Here's the drawing with two shaded views (mm, measured from the low corner). I have some questions. A direction names the side the tool comes from. Round coordinates to 2 decimals unless told otherwise and drop trailing zeros. Loops run counter-clockwise (first coordinate to the right, second up) from the corner with the lowest first, then second, coordinate; pieces in that order, holes last. Notation, with made-up numbers: (57.25, -10) -> (110.25, -10) arc R23 cw to (110.25, 9) -> close; hole circle Ø11 at (48, 64.5). An arc over 180 degrees is marked (long way). Use a Markdown table: item, result.
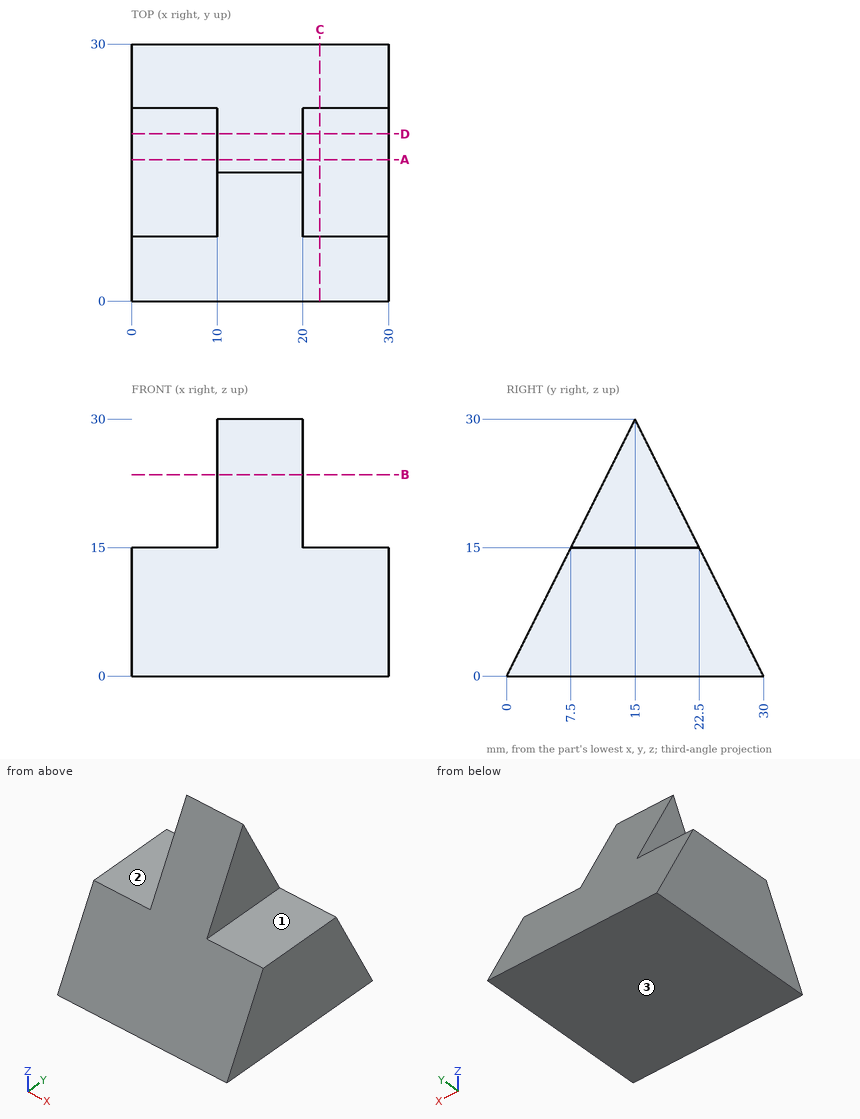
1. I want a section at A-A (y = 16.5). Please give me the cut outline in (x, z), plus the area to 3 significant figures.
Answer sheet:
| item | result |
|---|---|
| outline | (0, 0) -> (30, 0) -> (30, 15) -> (20, 15) -> (20, 27) -> (10, 27) -> (10, 15) -> (0, 15) -> close |
| area | 570 mm² |
2. Which directions (+Z, -Z, +X, -X, +Y, -Y) give clear straight access to the entire face, cutting with the end or side of a thin tool? Please do the marked faces 1, 2 and 3.
Answer sheet:
| item | result |
|---|---|
| face 1 | +Z, +X, +Y, -Y |
| face 2 | +Z, -X, +Y, -Y |
| face 3 | -Z, +X, -X, +Y, -Y |
3. Will these pins go through, and if not, where does the flat tip stop? pin 1 Ø3 at (x, y) = (14, 10) entering from +Z; pin 2 Ø12 at (x, z) = (9.5, 17) entering from +Y; pin 3 Ø3 at (x, y) = (5.5, 15) entering from +Z.
Answer sheet:
| item | result |
|---|---|
| pin 1 | stops at z = 23 |
| pin 2 | stops at y = 24.5 |
| pin 3 | stops at z = 15 |
4. I want a section at D-D (y = 19.5). Please give me the cut outline in (x, z), plus the area to 3 significant figures.
Answer sheet:
| item | result |
|---|---|
| outline | (0, 0) -> (30, 0) -> (30, 15) -> (20, 15) -> (20, 21) -> (10, 21) -> (10, 15) -> (0, 15) -> close |
| area | 510 mm² |
5. I want a section at C-C (x = 22). Please give me the cut outline in (y, z).
Answer sheet:
| item | result |
|---|---|
| outline | (0, 0) -> (30, 0) -> (22.5, 15) -> (7.5, 15) -> close |
6. I want a section at B-B (z = 23.5). Please give me the cut outline in (x, y), plus the area to 3 significant figures.
Answer sheet:
| item | result |
|---|---|
| outline | (10, 11.75) -> (20, 11.75) -> (20, 18.25) -> (10, 18.25) -> close |
| area | 65.0 mm² |
7. I need wall thicknesses on line 1 (Z direction, x = 8, y = 8); line 2 (Z direction, x = 2.25, y = 24.25); line 3 (Y direction, x = 5.5, z = 12). Which ranges of each line are inside material? Lowest first, please.
Answer sheet:
| item | result |
|---|---|
| line 1 | z = 0 to 15 |
| line 2 | z = 0 to 11.5 |
| line 3 | y = 6 to 24 |
